CAD build for the part. Positions are in the model's coordinates, mm. A direction names the side the tool comes from. Round coordinates to 2 decimals unless told otherwise and drop trailing zeros. Write each loop counter-clockwise with the first axis right and the second up, starting at its lowest first coordinate (ties: lowest second). Pieces come first, ordered by that corner, then holes. Notation, with made-up numbers: (85, 29.5) - (129, 29.5) arc R30 ccw to (129, 58.5) - close; hole circle Ø1 at (-39, 83). An arc over 180 degrees is marked (long way). Answer in a Markdown table with one row per item.
```python
from build123d import *

# Parameters (mm, degrees)
BOSS_EXTRUDE1_DEPTH       = 18
SKETCH3_W                 = 11.692277346
SKETCH3_H                 = 2
BOSS_EXTRUDE2_DEPTH       = 7
SKETCH4_W                 = 11.7
SKETCH4_H                 = 2
BOSS_EXTRUDE3_DEPTH       = 7
F_3_0MM_DOWEL_HOLE1_D     = 3
F_3_0MM_DOWEL_HOLE1_DEPTH = 12
F_3_0MM_DOWEL_HOLE1_TIP   = 0.901290929


with BuildPart() as part:
    # Sketch2 → Boss-Extrude1 (new body)
    with BuildSketch(Plane.XY):
        with BuildLine():
            Line((-9.25, 0), (-9.25, 9.5))
            ThreePointArc((-9.25, 9.5), (-8.664213562, 10.914213562), (-7.25, 11.5))
            Line((-7.25, 11.5), (7.25, 11.5))
            ThreePointArc((7.25, 11.5), (8.664213562, 10.914213562), (9.25, 9.5))
            Line((9.25, 9.5), (9.25, 0))
            Line((9.25, 0), (6.25, 0))
            Line((6.25, 0), (6.25, 10))
            Line((6.25, 10), (-6.25, 10))
            Line((-6.25, 10), (-6.25, 0))
            Line((-6.25, 0), (-9.25, 0))
        make_face()
    extrude(amount=BOSS_EXTRUDE1_DEPTH)

    # Sketch3 → Boss-Extrude2 (add)
    with BuildSketch(Plane(origin=(9.25, 0, 0), x_dir=(0, 0, -1), z_dir=(1, 0, 0))):
        with Locations((-9, 1)):
            Rectangle(SKETCH3_W, SKETCH3_H)
    extrude(amount=BOSS_EXTRUDE2_DEPTH)

    # Sketch4 → Boss-Extrude3 (add)
    with BuildSketch(Plane.ZY.offset(9.25)):
        with Locations((9, 1)):
            Rectangle(SKETCH4_W, SKETCH4_H)
    extrude(amount=BOSS_EXTRUDE3_DEPTH)

    # Ø3.0mm Dowel Hole1
    with Locations(Plane.XZ):
        with Locations((12.75, 9), (-12.75, 9)):
            Hole(F_3_0MM_DOWEL_HOLE1_D / 2, depth=F_3_0MM_DOWEL_HOLE1_DEPTH)
            with Locations((0, 0, -(F_3_0MM_DOWEL_HOLE1_DEPTH + F_3_0MM_DOWEL_HOLE1_TIP / 2))):  # 118° drill point
                Cone(0, F_3_0MM_DOWEL_HOLE1_D / 2, F_3_0MM_DOWEL_HOLE1_TIP, mode=Mode.SUBTRACT)


solid = part.part
```
Q1. Saw through at D-D on z = 4. List the corners of the cut face in (x, y).
Computed:
| item | result |
|---|---|
| outline | (-16.25, 0) - (-6.25, 0) - (-6.25, 10) - (6.25, 10) - (6.25, 0) - (16.25, 0) - (16.25, 2) - (9.25, 2) - (9.25, 9.5) arc R2 ccw to (7.25, 11.5) - (-7.25, 11.5) arc R2 ccw to (-9.25, 9.5) - (-9.25, 2) - (-16.25, 2) - close |
Q2. Saw through at B-B on x = 12.75. List the corners of the cut face in (y, z), then the cut area to 3 significant figures.
Computed:
| item | result |
|---|---|
| outline | (0, 3.15) - (2, 3.15) - (2, 7.5) - (0, 7.5) - close; (0, 10.5) - (2, 10.5) - (2, 14.85) - (0, 14.85) - close |
| area | 17.4 mm2 |
Q3. Flat gauge pins, fed straight in: pin 1 (3 mm diameter, centred on y = 7, z = 6, fed in from -X); pin 2 (7.5 mm diameter, centred on x = 14, z = 7, fed in from +Y); pin 3 (1.8 mm diameter, centred on x = -12.75, z = 9, fed in from +Y); pin 4 (10 mm diameter, centred on x = 0.5, z = 5.5, fed in from -Y). Where does each tip first touch, or does it go through?
Computed:
| item | result |
|---|---|
| pin 1 | stops at x = -9.25 |
| pin 2 | stops at y = 2 |
| pin 3 | passes through |
| pin 4 | stops at y = 10 |
Q4. Drill centre lines: line 1 (Z direction, x = -12.75, y = 0.8); line 2 (X direction, y = 9.25, z = 13); line 3 (Y direction, x = 0.5, z = 17.25). Where is each one in solid material? Low to high.
Computed:
| item | result |
|---|---|
| line 1 | z = 3.15 to 7.5, 10.5 to 14.85 |
| line 2 | x = -9.25 to -6.25, 6.25 to 9.25 |
| line 3 | y = 10 to 11.5 |
Q5. Saw through at A-A on z = 9. List the corners of the cut face in (x, y).
Computed:
| item | result |
|---|---|
| outline | (-16.25, 0) - (-14.25, 0) - (-14.25, 2) - (-16.25, 2) - close; (-11.25, 0) - (-6.25, 0) - (-6.25, 10) - (6.25, 10) - (6.25, 0) - (11.25, 0) - (11.25, 2) - (9.25, 2) - (9.25, 9.5) arc R2 ccw to (7.25, 11.5) - (-7.25, 11.5) arc R2 ccw to (-9.25, 9.5) - (-9.25, 2) - (-11.25, 2) - close; (14.25, 0) - (16.25, 0) - (16.25, 2) - (14.25, 2) - close |
Q6. 3-axis set-ups, long thin cutter, end or side, ignore diameter. For faces 1 (the flat face through (-13, 1, 14.85)), 2 (the flat face through (-13, 1, 3.15)), 3 (the flat face through (6.25, 5, 9)): which of +Z, -Z, +X, -X, +Y, -Y reach the whole face in a straight line?
Computed:
| item | result |
|---|---|
| face 1 | +Z, -X, +Y, -Y |
| face 2 | -Z, -X, +Y, -Y |
| face 3 | +Z, -Z, -Y |
Q7. Saw through at C-C on y = 9. List the corners of the cut face in (x, z).
Computed:
| item | result |
|---|---|
| outline | (-9.25, 0) - (-6.25, 0) - (-6.25, 18) - (-9.25, 18) - close; (6.25, 0) - (9.25, 0) - (9.25, 18) - (6.25, 18) - close |
